```python
from build123d import *

# Parameters (mm, degrees)
SKETCH1_R               = 2.5
BOSS_EXTRUDE1_DEPTH     = 18
SKETCH3_W               = 1
SKETCH3_H               = 0.5
BOSS_EXTRUDE2_DEPTH     = 5
CUT_EXTRUDE1_DEPTH      = 4
CUT_EXTRUDE1_DEPTH_BACK = 4
CUT_EXTRUDE2_DEPTH      = 34


with BuildPart() as part:
    # Sketch1 → Boss-Extrude1 (new body)
    with BuildSketch(Plane(origin=(0, 0, 0), x_dir=(1, 0, 0), z_dir=(0, 1, 0))):
        with Locations(Location((0, 0, 0), (0, 0, 270))):
            Circle(SKETCH1_R)
    extrude(amount=BOSS_EXTRUDE1_DEPTH)

    # Sketch3 → Boss-Extrude2 (add)
    with BuildSketch(Plane(origin=(0, 18, 0), x_dir=(1, 0, 0), z_dir=(0, 1, 0))):
        with Locations((0, 2.699489743)):
            Rectangle(SKETCH3_W, SKETCH3_H)
    extrude(amount=-BOSS_EXTRUDE2_DEPTH)

    # Sketch5 → Cut-Extrude1 (cut, two sides: drawn at the far end of the back side and taken through both)
    with BuildSketch(Plane.XY.offset(-CUT_EXTRUDE1_DEPTH_BACK)):
        Polygon((2.5, 14.4), (1.3, 9.721539031), (2.5, 9.4), align=None)
    extrude(amount=CUT_EXTRUDE1_DEPTH + CUT_EXTRUDE1_DEPTH_BACK, mode=Mode.SUBTRACT)

    # Sketch4 → Cut-Extrude2 (cut)
    with BuildSketch(Plane.XZ):
        with BuildLine():
            Line((-0.519059892, -1.299038106), (0.519059892, -1.299038106))
            ThreePointArc((0.519059892, -1.299038106), (0.719059892, -1.245448267), (0.865470054, -1.099038106))
            Line((0.865470054, -1.099038106), (1.384529946, -0.2))
            ThreePointArc((1.384529946, -0.2), (1.438119785, 0), (1.384529946, 0.2))
            Line((1.384529946, 0.2), (0.865470054, 1.099038106))
            ThreePointArc((0.865470054, 1.099038106), (0.719059892, 1.245448267), (0.519059892, 1.299038106))
            Line((0.519059892, 1.299038106), (-0.519059892, 1.299038106))
            ThreePointArc((-0.519059892, 1.299038106), (-0.719059892, 1.245448267), (-0.865470054, 1.099038106))
            Line((-0.865470054, 1.099038106), (-1.384529946, 0.2))
            ThreePointArc((-1.384529946, 0.2), (-1.438119785, 0), (-1.384529946, -0.2))
            Line((-1.384529946, -0.2), (-0.865470054, -1.099038106))
            ThreePointArc((-0.865470054, -1.099038106), (-0.719059892, -1.245448267), (-0.519059892, -1.299038106))
        make_face()
    extrude(amount=-CUT_EXTRUDE2_DEPTH, mode=Mode.SUBTRACT)


solid = part.part
```
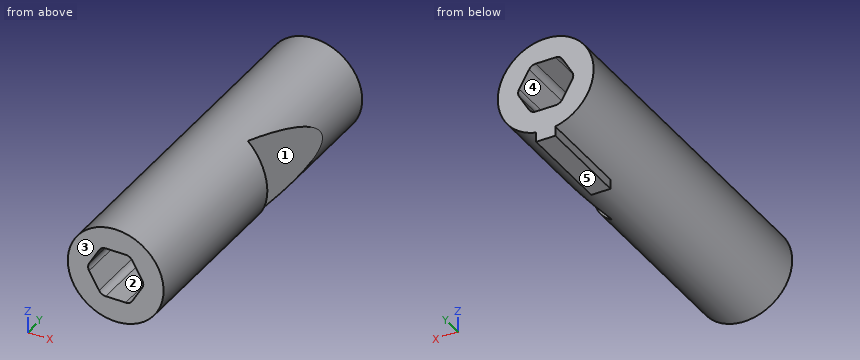
Source: CAD feature listing. Evaluate the final solid. Frame: model axes, mm. Face numbers are marked on the shaded views. A direction names the side the tool comes from. Give positions to 0.01 mm unless a question says otherwise; leave off trailing zeros. Loops run counter-clockwise (first coordinate to the right, second up) from the corner with the lowest first, then second, coordinate; pieces in that order, holes last. Notation, with made-up numbers: (18, 74.5) - (52, 74.5) arc R21 ccw to (52, 93.5) - close; hole circle Ø2 at (89.5, -25.75). An arc over 180 degrees is marked (long way). Use CSV: the item, a comma, the result in double quotes. Start each with the question number.
1. Section B-B (x = 0). Output: boundary loops of the cut face in (y, z).
2. Draft query along Y for the marked faces 1, 2 and 3. Return one class per face: +Y half, -Y half, draft (parallel to the pull), parting line (faces both ways), or undercut.
3. Pin query (flat end, axial travel): pin 1 (0.5 mm diameter, centred on x = 0, y = 5, fed in from -Z); pin 2 (0.6 mm diameter, centred on y = 15.5, z = -2.5, fed in from +X). Return the tip coordinate at first contact, or that it passes through.
4. Section C-C (z = -0.9). Output: boundary loops of the cut face in (x, y), then the cut area to 3 significant figures.
5. Section D-D (z = 0). Output: boundary loops of the cut face in (x, y).
6. Section A-A (y = 16.5). Output: boundary loops of the cut face in (x, z), then the cut area to 3 significant figures.
7. Reachability of the marked faces 4 and 5 from +Z, -Z, +X, -X, +Y, -Y: full face, straight path, thin tool, end or side. Return the list, or none.
8. Ray query, L1, parallel to X at y = 9.25, z = -0.05; L2, parallel to Z at x = -1.2, y = 7.75; L3, parallel to X at y = 7.25, z = -1.1 (3 decimals). Return the intervals inside material, ascending.
Response:
1,outline,"(0, -2.5) - (13, -2.5) - (13, -2.95) - (18, -2.95) - (18, -1.3) - (0, -1.3) - close; (0, 1.3) - (18, 1.3) - (18, 2.5) - (0, 2.5) - close"
2,face 1,"undercut"
2,face 2,"draft"
2,face 3,"-Y half"
3,pin 1,"z = -2.5"
3,pin 2,"x = 1.19"
4,outline,"(-2.33, 0) - (-0.98, 0) - (-0.98, 18) - (-2.33, 18) - close; (0.98, 0) - (2.33, 0) - (2.33, 9.44) - (1.3, 9.72) - (2.33, 13.75) - (2.33, 18) - (0.98, 18) - close"
4,area,"46.5 mm²"
5,outline,"(-2.5, 0) - (-1.44, 0) - (-1.44, 18) - (-2.5, 18) - close; (1.44, 0) - (2.5, 0) - (2.5, 9.4) - (1.44, 9.68) - close; (1.44, 10.26) - (2.5, 14.4) - (2.5, 18) - (1.44, 18) - close"
6,outline,"(-0.5, -2.95) - (0.5, -2.95) - (0.5, -2.45) arc R2.5 ccw (long way) to (-0.5, -2.45) - close; hole (-1.38, -0.2) - (-0.87, -1.1) arc R0.4 ccw to (-0.52, -1.3) - (0.52, -1.3) arc R0.4 ccw to (0.87, -1.1) - (1.38, -0.2) arc R0.4 ccw to (1.38, 0.2) - (0.87, 1.1) arc R0.4 ccw to (0.52, 1.3) - (-0.52, 1.3) arc R0.4 ccw to (-0.87, 1.1) - (-1.38, 0.2) arc R0.4 ccw to start"
6,area,"14.3 mm²"
7,face 4,"+Y, -Y"
7,face 5,"-Z, +X, -X, +Y, -Y"
8,L1,"-2.5 to -1.43, 1.43 to 2.5"
8,L2,"-2.19 to -0.52, 0.52 to 2.19"
8,L3,"-2.245 to -0.865, 0.865 to 2.245"
